Geometry: final body of the model. Coordinates: model frame, mm. A direction names the side the tool comes from. Give positions to 0.01 mm unless a question says otherwise; leave off trailing zeros. Loops run counter-clockwise (first coordinate to the right, second up) from the corner with the lowest first, then second, coordinate; pieces in that order, holes last. Notation, with made-up numbers: (34.5, 12) -> (56.5, 12) arc R31 cw to (56.5, 46) -> close; hole circle Ø11 at (30.25, 87). An arc over 180 degrees is marked (long way). Answer in a Markdown table with one row per item. Add a question column.
1) First-contact query: P1, Ø5, axis at x = -190.5, y = 122.5, coming from the +Z side. Flat tip, straight axial feed; report the tip coordinate or a pass-through.
2) Section query C-C (y = 121.5). Return the cut outline in (x, z), plus the area to 3 significant figures.
3) Access query for faces 1 (the flat face through (-192.25, 119.6, -0.9)), 2 (the flat face through (-192.088, 119.852, -0.756)). Directions: +Z, -Z, +X, -X, +Y, -Y. A direction counts if a zero-diameter tool reaches every point of the face in a straight line with its end or side. Return the directions, or none.
4) Section query A-A (z = -0.5). Return the cut outline in (x, y).
5) Line query: line 1 (X direction, y = 120, z = -1.05); line 2 (X direction, y = 121.75, z = -0.95); line 3 (Y direction, x = -193.25, z = -0.6). Output: solid intervals per line, ascending. Write a range as from..to.
6) Section query B-B (x = -195.5). Return the cut outline in (y, z).
```python
from build123d import *

# Parameters (mm, degrees)
BOX123_W               = 0.8
BOX123_H               = 15
BOX123_DEPTH           = 0.8
BOX124_W               = 0.8
BOX124_H               = 15
BOX124_DEPTH           = 0.8
CUT065_PLACEMENT_ANGLE = 58


with BuildPart() as cubo123:
    # Box123 → Box123 (new body)
    with BuildSketch(Plane.XY):
        with Locations((0.4, 7.5)):
            Rectangle(BOX123_W, BOX123_H)
    extrude(amount=BOX123_DEPTH)


with BuildPart() as obj1:
    # Box124 → Box124 (new body)
    with BuildSketch(Plane(origin=(0.3, 0, 0.3), x_dir=(1, 0, 0), z_dir=(0, 0, 1))):
        with Locations((0.4, 7.5)):
            Rectangle(BOX124_W, BOX124_H)
    extrude(amount=BOX124_DEPTH)

    # Cut065: cut Cubo123
    add(cubo123.part, mode=Mode.SUBTRACT)


with BuildPart() as obj1_1:
    # Cut065 placement: moved
    add(obj1.part.moved(Location((-186.4, 115, -1.45))).rotate(Axis((-186.4, 115, -1.45), (0, 0, 1)), CUT065_PLACEMENT_ANGLE))


solid = obj1_1.part
```
Evaluation:
| question | item | result |
|---|---|---|
| 1 | P1 | through |
| 2 | outline | (-196.24, -0.65) -> (-195.29, -0.65) -> (-195.29, -1.15) -> (-194.73, -1.15) -> (-194.73, -0.35) -> (-196.24, -0.35) -> close |
| 2 | area | 0.736 mm² |
| 3 | face 1 | -Z, -X, -Y |
| 3 | face 2 | +Z, -Z, +X, +Y |
| 4 | outline | (-198.96, 123.2) -> (-186.24, 115.25) -> (-185.82, 115.93) -> (-198.54, 123.88) -> close |
| 5 | line 1 | -192.89..-192.33 |
| 5 | line 2 | -195.69..-195.13 |
| 5 | line 3 | 119.63..120.58 |
| 6 | outline | (121.04, -0.65) -> (121.63, -0.65) -> (121.63, -1.15) -> (121.98, -1.15) -> (121.98, -0.35) -> (121.04, -0.35) -> close |
